Autodesk Inventor part; units mm, degrees
ref_plane "BackFace" through (0, -1, 0) normal (0, 1, 0) x (-1, 0, 0)
ref_plane "BottomFace" through (0, -4.2, 0) normal (0, 1, 0) x (-1, 0, 0)
ref_plane "YZ Plane" through (0, 0, 0) normal (1, 0, 0) x (0, 1, 0)
ref_plane "BackFace" through (0, -1, 0) normal (0, 1, 0) x (-1, 0, 0)
ref_plane "BottomFace" through (0, -4.2, 0) normal (0, 1, 0) x (-1, 0, 0)
sketch "FemaleOutline" plane through (0, 0, 0) normal (0, 1, 0) x (-1, 0, 0)
  line L0 (0, -26.6) -> (0, 26.6)
  line L1 (-3, 0) -> (18, 0)
  line L2 (0.4908, -4.8956) -> (9.5, -6.65)
  line L3 (9.5, -6.65) -> (9.5, 6.65)
  line L4 (9.5, 6.65) -> (0.4908, 4.8956)
  line L5 (0, -19) -> (0, -5.3)
  line L6 (0, 5.3) -> (0, 19)
  line L7 (2.4, -6.9) -> (11.5, -6.9)
  line L8 (11.5, -6.9) -> (11.5, 6.9)
  line L9 (11.5, 6.9) -> (2.4, 6.9)
  line L10 (2.4, -6.9) -> (0, -9.3)
  line L11 (2.4, 6.9) -> (0, 9.3)
  line L12 (15, -16) -> (15, 16)
  line L13 (15, 16) -> (0, 19)
  line L14 (15, -16) -> (0, -19)
  line L15 (0.4908, 4.8956) -> (0, 5.3)
  line L16 (0.4908, -4.8956) -> (0, -5.3)
  point P0 (0, 0)
  point P1 (0, -4.8)
  point P2 (0, 4.8)
  point P3 (0, 9.3)
  point P4 (0, 4.8)
  point P5 (0, -4.8)
  point P6 (0, -9.3)
  point P7 (0, -5.3)
  point P8 (0, 5.3)
  dimension "d3" = 13.3
  dimension "d5" = 9.6
  dimension "d14" = 2
  dimension "d63" = 2.4
  dimension "d64" = 18.6
  dimension "d65" = 15
  dimension "d74" = 38
  dimension "d75" = 3
  dimension "d93" = 9.5
  dimension "d94" = 2.4
  dimension "d95" = 0.5
  dimension "d96" = 0.5
  dimension "d97" = 0.5
  dimension "d98" = 0.5
sketch "MaleOutline" plane through (0, 0, 0) normal (0, 1, 0) x (-1, 0, 0)
  line L0 (0, -4.7) -> (-8.5097, -6.4019)
  line L1 (-9, -6) -> (-9, 6)
  line L2 (-8.5097, 6.4019) -> (0, 4.7)
  line L3 (0, -19) -> (0, -4.7)
  line L4 (0, 4.7) -> (0, 19)
  line L5 (2.4, -1.7725) -> (-6.6, -3.5725)
  line L6 (-6.6, -3.5725) -> (-6.6, 3.5725)
  line L7 (-6.6, 3.5725) -> (2.4, 1.7725)
  line L8 (2.4, -6.9) -> (2.4, -1.7725)
  line L9 (2.4, 1.7725) -> (2.4, 6.9)
  line L10 (2.4, -6.9) -> (0, -9.3)
  line L11 (2.4, 6.9) -> (0, 9.3)
  line L12 (15, -16) -> (15, 16)
  line L13 (15, 16) -> (0, 19)
  line L14 (15, -16) -> (0, -19)
  line L15 (0, -26.6) -> (0, 26.6)
  line L16 (-13.8, 0) -> (19.8, 0)
  line L17 (-8.5097, -6.4019) -> (-9, -6)
  line L18 (-9, 6) -> (-8.5097, 6.4019)
  point P0 (-9, -6.5)
  point P1 (-9, 6.5)
  dimension "d99" = 9
  dimension "d100" = 13
  dimension "d101" = 9.4
  dimension "d102" = 2.4
  dimension "d103" = 2.4
  dimension "d104" = 2.4
  dimension "d105" = 2.4
  dimension "d106" = 2.4
  dimension "d107" = 18.6
  dimension "d109" = 38
  dimension "d110" = 3
  dimension "d120" = 15
  dimension "d128" = 0.5
  dimension "d129" = 0.5
  dimension "d130" = 0.5
  dimension "d131" = 0.5
sketch "DipOutline" plane through (0, -1, 0) normal (0, 1, 0) x (-1, 0, 0)
  line L0 (0, -120.0212) -> (0, 93.8212)
  line L1 (-3, 0) -> (18, 0)
  line L2 (0, 19) -> (15, 16)
  line L3 (15, 16) -> (15, -16)
  line L4 (15, -16) -> (0, -19)
  line L5 (0, -19) -> (0, 19)
  line L6 (0, 19) -> (0, 4.7)
  line L7 (10.95, -6.3) -> (14.95, -6.3)
  line L8 (14.95, -6.3) -> (14.95, -2.6)
  line L9 (14.95, -2.6) -> (10.95, -2.6)
  line L10 (10.95, -2.6) -> (10.95, -6.3)
  line L11 (14.95, -15.85) -> (14.95, -10.35)
  arc A0 (14.95, -10.35) -> (0, -8.95) centre (0, -89.4723) ccw
  arc A1 (0, -17.25) -> (14.95, -15.85) centre (0, 63.2723) ccw
  line L12 (9.5, 0) -> (9.5, -6.9)
  line L13 (9.5, -6.9) -> (0, -6.9)
  line L14 (0, -8.45) -> (0.5, -8.9516)
  line L15 (0, -17.75) -> (0.5, -17.2484)
  point P0 (0, -17.25)
  point P1 (15, 0)
  point P2 (0, 0)
  point P3 (0, -8.95)
  dimension "d133" = 15
  dimension "d134" = 38
  dimension "d135" = 3
  dimension "d146" = 3.7
  dimension "d147" = 6.3
  dimension "d148" = 2.6
  dimension "d151" = 14.95
  dimension "d152" = 4
  dimension "d153" = 5.5
  dimension "d154" = 8.3
  dimension "d155" = 17.25
  dimension "d160" = 6.9
  dimension "d161" = 9.5
  dimension "d196" = 0.5
  dimension "d197" = 0.5
  dimension "d198" = 0.5
  dimension "d199" = 0.5
sketch "DipSupport" plane through (0, -4.2, 0) normal (0, 1, 0) x (-1, 0, 0)
  line L0 (0, -20.94) -> (0, 3.49)
  line L1 (-5.0794, 0) -> (17.4132, 0)
  line L2 (-1.8662, -13.1) -> (-0.8497, -13.1)
  line L3 (0, -9.95) -> (0, -16.25)
  line L4 (0, -16.25) -> (0.6, -16.25)
  line L5 (0.6, -16.25) -> (0.6, -15.5)
  line L6 (0.6, -14.8486) -> (0.6, -13.35)
  line L7 (0.6, -13.35) -> (13.117, -13.35)
  line L8 (13.117, -13.35) -> (13.4421, -13.9987)
  line L9 (13.4421, -13.9987) -> (0.6, -14.8486)
  line L10 (0.6, -12.85) -> (13.117, -12.85)
  line L11 (13.117, -12.85) -> (13.4421, -12.2013)
  line L12 (13.4421, -12.2013) -> (0.6, -11.3514)
  line L13 (0.6, -11.3514) -> (0.6, -12.85)
  line L14 (0, -9.95) -> (0.6, -9.95)
  line L15 (0.6, -9.95) -> (0.6, -10.7)
  line L16 (0, -9.95) -> (0, -8.75)
  line L17 (0, -8.75) -> (0.3, -8.75)
  line L18 (0.3, -8.75) -> (0.6, -9.05)
  line L19 (0.6, -9.05) -> (0.6, -9.95)
  line L20 (0, -16.25) -> (0, -17.45)
  line L21 (0.3, -17.45) -> (0.6, -17.15)
  line L22 (0.6, -17.15) -> (0.6, -16.25)
  line L23 (0, -17.45) -> (0.3, -17.45)
  line L24 (0.6, -15.5) -> (14.2, -14.6)
  line L25 (14.2, -14.6) -> (14.2, -13.9486)
  line L26 (14.2, -13.9486) -> (13.9, -13.35)
  line L27 (13.9, -13.35) -> (13.9, -12.85)
  line L28 (13.9, -12.85) -> (14.2, -12.2514)
  line L29 (14.2, -12.2514) -> (14.2, -11.6)
  line L30 (14.2, -11.6) -> (0.6, -10.7)
  line L31 (0, -9.95) -> (0, -8.75)
  line L32 (0, -16.25) -> (0, -17.45)
  point P0 (0, 0)
  point P1 (0, -17.25)
  point P2 (0, -8.95)
  dimension "d169" = 0.5
  dimension "d171" = 4.8
  dimension "d181" = 4.15
  dimension "d182" = 4.15
  dimension "d183" = 0.2
  dimension "d184" = 1
  dimension "d185" = 0.3
  dimension "d186" = 0.6
  dimension "d187" = 45
  dimension "d188" = 14.2
  dimension "d189" = 3
  dimension "d190" = 0.65
  dimension "d191" = 0.3
  dimension "d193" = 0.7
extrude "Female1" [suppressed]
extrude "Female2" [suppressed]
chamfer "FemaleC" [suppressed]
extrude "FemaleFill" [suppressed]
extrude "Male1" add sketch "MaleOutline" along normal mid plane 8.4 separate body contours L15 L5 L8 L10 L3 | L0 L17 L1 L16 L6 L5 L15 | L1 L18 L2 L15 L7 L6 L16 | L15 L4 L11 L9 L7
extrude "Male2" add sketch "MaleOutline" along normal mid plane 2 contours L10 L8 L5 L15 L16 L12 L14 L3 | L5 L6 L16 L15 | L16 L6 L7 L15 | L15 L7 L9 L11 L4 L13 L12 L16
chamfer "MaleC" distance 0.7 angle 45 10 edges at (2.1, 1, -2.6725) (2.1, 1, 2.6725) (6.6, 1, 0) (2.1, -1, 2.6725) (6.6, -1, 0) (2.1, -1, -2.6725) (-2.4, -1, 4.3362) (-2.4, -1, -4.3362) (-2.4, 1, 4.3362) (-2.4, 1, -4.3362)
extrude "MaleFill" [suppressed]
extrude "JointDip" [suppressed]
extrude "JointDipSup1" [suppressed]
extrude "JointDipSup2" [suppressed]
mirror "JointDipM" [suppressed]
mirror "JointDipSupM" [suppressed]
sketch "PrintTab" plane through (0, -4.2, 0) normal (0, 1, 0) x (-1, 0, 0)
  line L0 (0, -30.8) -> (0, 30.8)
  line L1 (-10.4076, 0) -> (1.7346, 0)
  line L2 (0, -19) -> (0, -17)
  line L3 (0, 17) -> (0, 19)
  line L4 (0, 19) -> (-0.8, 19)
  line L5 (0, 17) -> (-0.8, 17)
  line L6 (0, -17) -> (-0.8, -17)
  line L7 (0, -19) -> (-0.8, -19)
  line L8 (-0.8, -19) -> (-0.8, -17)
  line L9 (-0.8, 17) -> (-0.8, 19)
  arc A0 (-0.8, 19) -> (-0.8, 17) centre (-4.673, 18) ccw
  arc A1 (-0.8, -17) -> (-0.8, -19) centre (-4.673, -18) ccw
  point P0 (0, 0)
  dimension "d208" = 2
  dimension "d209" = 38
  dimension "d216" = 0.8
  dimension "d217" = 4
extrude "PrintTab1" [suppressed]
extrude "PrintTab2" [suppressed]
equation "\"d19\" = RailHeight"
equation "\"rib\" = 0.65"
equation "\"gap\" = 0.2"
equation "\"d118\" = 0"
equation "\"d143\" = 0"
equation "\"d178\" = 0.5"
properties part number "MaleDoubleSide" material "ABS プラスチック"
Can you work these out from the model? Positions are in its coordinate system, mm. A direction names the side the tool comes from. Coordinates: 2 decimals unless noted, no trailing zeros. Write each loop counter-clockwise with the first axis right and the second up, starting at its lowest first coordinate (ties: lowest second). Pieces come first, ordered by that corner, then holes. Notation, with made-up numbers: (77.25, 66) -> (135.25, 66) arc R27 cw to (135.25, 92) -> close; hole circle Ø3 at (-18.75, -22). An arc over 180 degrees is marked (long way). Answer as CSV lines item,"result".
1) If we mould it in two halves opening along X, with no side actions, what happens to faces 5 (the flat face through (-2.4, 3, 4)), 6 (the flat face through (6.6, 3, 0)), 7 (the flat face through (9, 0, 0))? For each: +X half, -X half, draft (parallel to the pull), parting line (faces both ways), or undercut.
Check result:
face 5,"-X half"
face 6,"undercut"
face 7,"+X half"
2) If we section it at C-C on z = 0: Please give me the cut outline in (x, y), then the cut area to 4 significant figures.
Check result:
outline,"(-15, -1) -> (5.9, -1) -> (6.6, -1.7) -> (6.6, -4.2) -> (9, -4.2) -> (9, 4.2) -> (6.6, 4.2) -> (6.6, 1.7) -> (5.9, 1) -> (-15, 1) -> close"
area,"63.85 mm²"
3) If we section it at A-A on z = 5.5: Please give me the cut outline in (x, y), then the cut area to 3 significant figures.
Check result:
outline,"(-15, -1) -> (-3.1, -1) -> (-2.4, -1.7) -> (-2.4, -4.2) -> (0, -4.2) -> (0, 4.2) -> (-2.4, 4.2) -> (-2.4, 1.7) -> (-3.1, 1) -> (-15, 1) -> close; (4, -4.2) -> (9, -4.2) -> (9, 4.2) -> (4, 4.2) -> close"
area,"87.8 mm²"
4) Will these pins go through, and if not, where does the flat tip stop? P1, Ø3, axis at y = 3.5, z = 3, coming from the -X side; P2, Ø1, axis at x = 3.5, y = 1, coming from the +Z side; P3, Ø1.5, axis at y = 0, z = 9.5, coming from the +X side.
Check result:
P1,"x = -2.4"
P2,"z = 5.5"
P3,"x = 0"
5) On a 3-axis mill with a long thin cutter (end or side, diameter ignored), from which of +Z, -Z, +X, -X, +Y, -Y can I reach the whole of each face in a straight line? I mean faces 1 (the flat face through (-1.2, 2.6, 8.1)), 2 (the flat face through (1.82, 1.345, -2.255)), 3 (the flat face through (-2.4, 3, -4)), 4 (the flat face through (-1.2, -2.6, 8.1)). Say none if no direction works.
Check result:
face 1,"+Z, -X, +Y"
face 2,"+Y"
face 3,"+Z, -Z, -X, +Y"
face 4,"+Z, -X, -Y"
6) If I drill on line 1 (Y direction, x = -13, z = 10.5); line 2 (Z direction, x = -0.75, y = 1.75); line 3 (Z direction, x = 0.75, y = -2), over which ranges is the centre line in solid material (lowest first)? Write a range as from..to.
Check result:
line 1,"-1..1"
line 2,"-8.55..-2.1, 2.1..8.55"
line 3,"-4.85..-2.4, 2.4..4.85"
7) If we section it at B-B on y = 3: Please give me the cut outline in (x, z), then the cut area to 3 significant figures.
Check result:
outline,"(-2.4, -6.9) -> (0, -9.3) -> (0, -4.7) -> (8.51, -6.4) -> (9, -6) -> (9, 6) -> (8.51, 6.4) -> (0, 4.7) -> (0, 9.3) -> (-2.4, 6.9) -> (-2.4, 1.77) -> (6.6, 3.57) -> (6.6, -3.57) -> (-2.4, -1.77) -> close"
area,"91.3 mm²"
8) If we section it at D-D on x = -7.5: Please give me the cut outline in (y, z).
Check result:
outline,"(-1, -17.5) -> (1, -17.5) -> (1, 17.5) -> (-1, 17.5) -> close"
